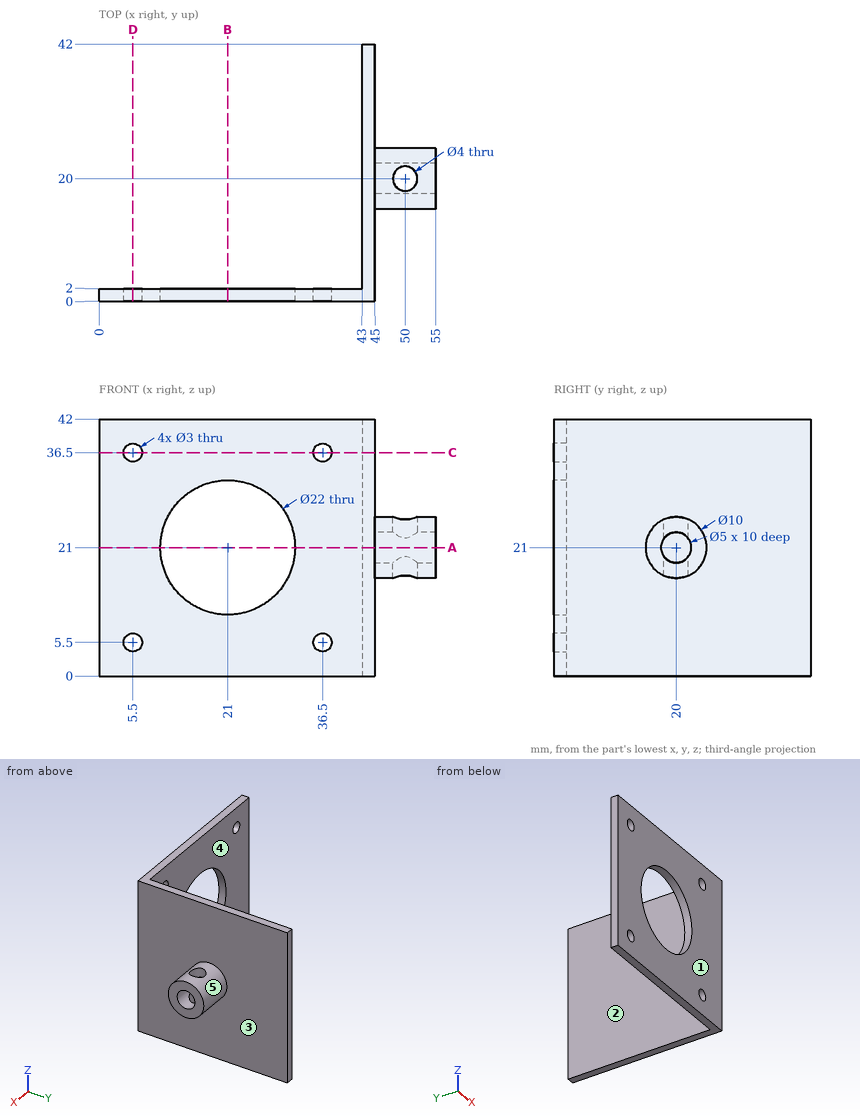
Source: three-view drawing plus pictorial views. Frame: mm from the lowest corner of the part. A direction names the side the tool comes from. Round coordinates to 2 decimals unless told otherwise and drop trailing zeros. Loops run counter-clockwise (first coordinate to the right, second up) from the corner with the lowest first, then second, coordinate; pieces in that order, holes last. Notation, with made-up numbers: (8, 27) -> (58, 27) arc R4 cw to (58, 31) -> close; hole circle Ø11 at (86.5, 71.25). An arc over 180 degrees is marked (long way). Use one line per item in the form item = value.
Item 1: Draft query along X for the marked faces 1, 2 and 3. Return one class per face: released by +X, released by -X, zero draft, split by the parting line, or undercut.
Evaluation:
face_1 = zero draft
face_2 = released by -X
face_3 = released by +X
Item 2: Material intervals for probe 1 along X at (y, z) = (1, 36.5); probe 2 along X at (y, z) = (20, 17.15); probe 3 along Y at (x, z) = (47.5, 21), sorted ascending.
Evaluation:
probe_1 = 0 to 4, 7 to 35, 38 to 45
probe_2 = 43 to 48, 52 to 55
probe_3 = 15 to 17.5, 22.5 to 25
Item 3: Cut plane D-D on x = 5.5. Output: boundary loops of the cut face in (y, z), then the cut area to 3 significant figures.
Evaluation:
outline = (0, 0) -> (2, 0) -> (2, 4) -> (0, 4) -> close; (0, 7) -> (2, 7) -> (2, 35) -> (0, 35) -> close; (0, 38) -> (2, 38) -> (2, 42) -> (0, 42) -> close
area = 72.0 mm2
Item 4: Cut plane B-B on x = 21. Output: boundary loops of the cut face in (y, z), then the cut area to 3 significant figures.
Evaluation:
outline = (0, 0) -> (2, 0) -> (2, 10) -> (0, 10) -> close; (0, 32) -> (2, 32) -> (2, 42) -> (0, 42) -> close
area = 40.0 mm2
Item 5: Contact query for flat-ended pins moving along their axis: pin 1 Ø3.5 at (x, y) = (50, 20) entering from -Z; pin 2 Ø12 at (y, z) = (31, 23) entering from -X; pin 3 Ø4.5 at (x, y) = (50, 20) entering from -Z. Output: stop coordinate, or through.
Evaluation:
pin_1 = through
pin_2 = 43
pin_3 = 16
Item 6: Access query for the marked faces 4 and 5. Directions: +Z, -Z, +X, -X, +Y, -Y. A direction counts if a zero-diameter tool reaches every point of the face in a straight line with its end or side. Return the directions, or none.
Evaluation:
face_4 = +Z, -Z, -X, +Y
face_5 = +X
Item 7: Cut plane C-C on z = 36.5. Output: boundary loops of the cut face in (x, y).
Evaluation:
outline = (0, 0) -> (4, 0) -> (4, 2) -> (0, 2) -> close; (7, 0) -> (35, 0) -> (35, 2) -> (7, 2) -> close; (38, 0) -> (45, 0) -> (45, 42) -> (43, 42) -> (43, 2) -> (38, 2) -> close
Item 8: Cut plane A-A on z = 21. Output: boundary loops of the cut face in (x, y), then the cut area to 3 significant figures.
Evaluation:
outline = (0, 0) -> (10, 0) -> (10, 2) -> (0, 2) -> close; (32, 0) -> (45, 0) -> (45, 15) -> (55, 15) -> (55, 17.5) -> (45, 17.5) -> (45, 22.5) -> (55, 22.5) -> (55, 25) -> (45, 25) -> (45, 42) -> (43, 42) -> (43, 2) -> (32, 2) -> close
area = 176 mm2
